```python
from build123d import *

# Parameters (mm, degrees)
F0_R     = 11
F1_DEPTH = 10
F2_R     = 5
F3_DEPTH = 25
F4_R     = 1
F5_DEPTH = 25


with BuildPart() as f1:
    # F0 (on Front) → F1 (new body)
    with BuildSketch(Plane.XZ):
        Circle(F0_R)
    extrude(amount=F1_DEPTH)

    # F2 (on face) → F3 (cut)
    with BuildSketch(Plane.XZ.offset(10)):
        Circle(F2_R)
    extrude(amount=-F3_DEPTH, mode=Mode.SUBTRACT)

    # F4 (on face) → F5 (cut)
    with BuildSketch(Plane.XZ.offset(10)):
        with Locations((-8, 0)):
            Circle(F4_R)
        with Locations((0, 8)):
            Circle(F4_R)
        with Locations((8, 0)):
            Circle(F4_R)
        with Locations((0, -8)):
            Circle(F4_R)
    extrude(amount=-F5_DEPTH, mode=Mode.SUBTRACT)


solid = f1.part
```
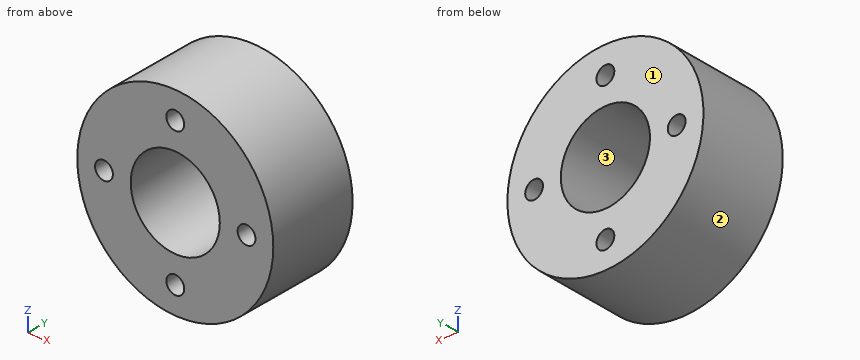
For this review, take the finished solid that the model builds, in its own axes (mm). Face numbers are marked on the shaded views. Round coordinates to 2 decimals unless told otherwise and drop trailing zeros. Write each loop counter-clockwise with the first axis right and the second up, starting at its lowest first coordinate (ties: lowest second). Pieces come first, ordered by that corner, then holes. Notation, with made-up numbers: (-35.75, 10) -> (-6.75, 10) arc R22 cw to (-6.75, 30) -> close; hole circle Ø11 at (-11.75, -18). An arc over 180 degrees is marked (long way). Use one line per item in the form item = value.
1) Clearance check with flat-ended pins moving along their axes: pin 1 (8 mm diameter, centred on x = 0, z = 0, fed in from +Y); pin 2 (2.5 mm diameter, centred on x = 8, z = 0, fed in from +Y); pin 3 (2 mm diameter, centred on x = -6, y = -3, fed in from +Z); pin 4 (5 mm diameter, centred on y = -1.5, z = 4, fed in from +X). State where each tip first meets the part, or that it passes through.
Found:
pin_1 = through
pin_2 = 0
pin_3 = 9.8
pin_4 = 10.9
2) Take a section at C-C, the plane x = 3. Write out the cut boundary in (y, z), and give its area (3 significant figures).
Found:
outline = (-10, -10.58) -> (0, -10.58) -> (0, -4) -> (-10, -4) -> close; (-10, 4) -> (0, 4) -> (0, 10.58) -> (-10, 10.58) -> close
area = 132 mm2
3) Mouldability with a two-part tool opening along X and no side actions: class the marked faces 1, 2 and 3 as +X half, -X half, draft (parallel to the pull), parting line (faces both ways), or undercut.
Found:
face_1 = draft
face_2 = parting line
face_3 = undercut
4) Take a section at A-A, the plane z = 4.25. Write out the cut boundary in (x, y).
Found:
outline = (-10.15, -10) -> (-2.63, -10) -> (-2.63, 0) -> (-10.15, 0) -> close; (2.63, -10) -> (10.15, -10) -> (10.15, 0) -> (2.63, 0) -> close
5) Take a section at B-B, the plane x = 0. Write out the cut boundary in (y, z), and give its area (3 significant figures).
Found:
outline = (-10, -11) -> (0, -11) -> (0, -9) -> (-10, -9) -> close; (-10, -7) -> (0, -7) -> (0, -5) -> (-10, -5) -> close; (-10, 5) -> (0, 5) -> (0, 7) -> (-10, 7) -> close; (-10, 9) -> (0, 9) -> (0, 11) -> (-10, 11) -> close
area = 80.0 mm2
6) To check wall thickness, follow L1, parallel to Z at x = 0, y = -3.75; L2, parallel to X at y = -8, z = -4.5; L3, parallel to X at y = -5.75, z = -0.5. State the ranges of each line that lie inside material, in increasing order. Write a range as from..to.
Found:
L1 = -11..-9, -7..-5, 5..7, 9..11
L2 = -10.04..-2.18, 2.18..10.04
L3 = -10.99..-8.87, -7.13..-4.97, 4.97..7.13, 8.87..10.99
7) Take a section at D-D, the plane y = -4. Write out the cut boundary in (x, z).
Found:
outline = circle Ø22 at (0, 0); hole circle Ø2 at (-8, 0); hole circle Ø10 at (0, 0); hole circle Ø2 at (0, -8); hole circle Ø2 at (0, 8); hole circle Ø2 at (8, 0)
